Design review of the part shown in the three views and the two pictorial views. Dimensions are in mm from the part's minimum x, y and z. A direction names the side the tool comes from. Coordinates: 2 decimals unless noted, no trailing zeros. Loops run counter-clockwise (first coordinate to the right, second up) from the corner with the lowest first, then second, coordinate; pieces in that order, holes last. Notation, with made-up numbers: (-27.5, 78) -> (16.5, 78) arc R22 ccw to (16.5, 108) -> close; hole circle Ø8 at (-15, 70.25). An arc over 180 degrees is marked (long way). One line per item, written item: value. Start each with the question number.
1. For probe 1 along Z at (x, y) = (12.5, 1.45) (3 decimals); probe 2 along Y at (x, z) = (7, 4.25); probe 3 along Z at (x, y) = (12.75, 3), list the stretches that pass through material, from the lowest coordinate up.
2. Add section B-B on z = 20. Write out the cut boundary in (x, y), plus the area to 3 significant figures.
3. Add section A-A on y = 5.05. Write out the cut boundary in (x, z), plus the area to 3 significant figures.
4. Machinability: for the marked faces 1 and 2, which of the approach directions +Z, -Z, +X, -X, +Y, -Y give a long, thin tool a straight path to every point of the face, cutting with its end or side? Answer none if there is none.
5. Add section C-C on x = 7.75. Write out the cut boundary in (y, z), plus the area to 3 significant figures.
6. Draft analysis for pull direction X (two halves, no side actions). For the marked faces 3, 4 and 5, state which applies: pulls with the +X half, pulls with the -X half, needs draft (parallel to the pull), parting line crosses it, or undercut.
7. Insertion check: pin 1 (3 mm diameter, centred on x = 16, y = 2, fed in from -Z); pin 2 (2 mm diameter, centred on x = 22, z = 15, fed in from -Y); pin 3 (3 mm diameter, centred on x = 17, y = 1, fed in from -Z). Each pin has a flat end and moves straight along its axis. Give the tip position at first contact, or say it passes through.
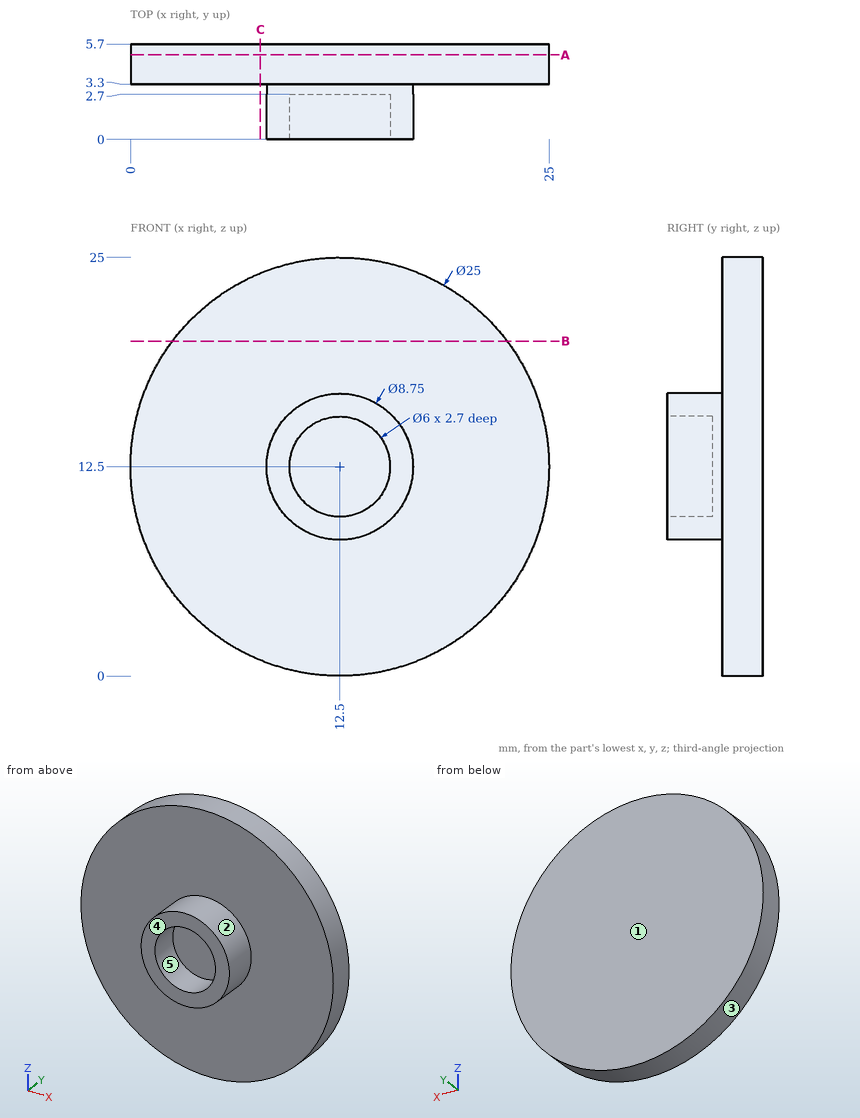
Worked answers:
1. probe 1: z = 8.125 to 9.5, 15.5 to 16.875
1. probe 2: y = 3.3 to 5.7
1. probe 3: z = 8.13 to 16.87
2. outline: (2.5, 3.3) -> (22.5, 3.3) -> (22.5, 5.7) -> (2.5, 5.7) -> close
2. area: 48.0 mm²
3. outline: circle Ø25 at (12.5, 12.5)
3. area: 491 mm²
4. face 1: +Z, -Z, +X, -X, +Y
4. face 2: -Y
5. outline: (3.3, 0.94) -> (5.7, 0.94) -> (5.7, 24.06) -> (3.3, 24.06) -> close
5. area: 55.5 mm²
6. face 3: parting line crosses it
6. face 4: needs draft
6. face 5: undercut
7. pin 1: stops at z = 0.31
7. pin 2: stops at y = 3.3
7. pin 3: stops at z = 9.32
